```python
from build123d import *

# Parameters (mm, degrees)
CROQUIS1_W              = 37.6
CROQUIS1_H              = 15
CROQUIS1_R              = 1.5
SALIENTE_EXTRUIR1_DEPTH = 2
CROQUIS2_W              = 2.997393123
CROQUIS2_H              = 15
SALIENTE_EXTRUIR2_DEPTH = 20
CROQUIS3_R              = 1.3
CORTAR_EXTRUIR1_DEPTH   = 20


with BuildPart() as part:
    # Croquis1 → Saliente-Extruir1 (new body)
    with BuildSketch(Plane(origin=(0, 0, 0), x_dir=(1, 0, 0), z_dir=(0, 1, 0))):
        Rectangle(CROQUIS1_W, CROQUIS1_H)
        with Locations(Location((14.3, -3.2, 0), (0, 0, 270))):
            Circle(CROQUIS1_R, mode=Mode.SUBTRACT)
        with Locations(Location((-14.3, -3.2, 0), (0, 0, 90))):
            Circle(CROQUIS1_R, mode=Mode.SUBTRACT)
    extrude(amount=SALIENTE_EXTRUIR1_DEPTH)

    # Croquis2 → Saliente-Extruir2 (add)
    with BuildSketch(Plane(origin=(0, 2, 0), x_dir=(1, 0, 0), z_dir=(0, 1, 0))):
        with Locations((-4.748696562, 0)):
            Rectangle(CROQUIS2_W, CROQUIS2_H)
        with Locations((4.748696562, 0)):
            Rectangle(CROQUIS2_W, CROQUIS2_H)
    extrude(amount=SALIENTE_EXTRUIR2_DEPTH)

    # Croquis3 → Cortar-Extruir1 (cut)
    with BuildSketch(Plane.ZY.offset(6.247393123)):
        with Locations((0.3, 16.669676255)):
            Circle(CROQUIS3_R)
        with Locations((0.3, 7.330323745)):
            Circle(CROQUIS3_R)
    extrude(amount=-CORTAR_EXTRUIR1_DEPTH, mode=Mode.SUBTRACT)


solid = part.part
```
CAD build for the part. Positions are in the model's coordinates, mm. A direction names the side the tool comes from. Round coordinates to 2 decimals unless told otherwise and drop trailing zeros. Loops run counter-clockwise (first coordinate to the right, second up) from the corner with the lowest first, then second, coordinate; pieces in that order, holes last. Notation, with made-up numbers: M 49,53.5 L 100,53.5 A16 cw 100,68.5 Z; hole C 25.5,38 d7. An arc over 180 degrees is marked long. Use a Markdown table: item, result. Add a question column.
(1) Pull direction X, two halves, no side cores. Call faces 1 (the face through (6.247, 12, 0)), 2 (the face through (0, 2, 0)), 3 (the face through (12.836, 0.986, 2.875)), 4 (the face through (-4.77, 8.426, 0.999)): +X half, -X half, draft (parallel to the pull), parting line (faces both ways), or undercut.
(2) Cut at A-A (z = 3.2). Give the cut face in (x, y).
(3) Which spindle directions (+Z, -Z, +X, -X, +Y, -Y) get a long thin tool onto all of the face, cutting with end or side? Do faces 5 (the face through (-6.247, 12, 0)), 6 (the face through (3.25, 12, 0)), 7 (the face through (12, 2, 0)). Say none if no direction does.
(4) Cut at B-B (y = 13.75). Give the cut face in (x, z), and give its area (3 significant figures).
(5) Flat gauge pins, fed straight in: pin 1 (3 mm diameter, centred on y = 7.33, z = 0.3, fed in from +X); pin 2 (5 mm diameter, centred on x = 14.3, z = 3.2, fed in from -Y); pin 3 (3.5 mm diameter, centred on y = 16.67, z = 0.3, fed in from -X). Where does each tip first touch, or does it go through?
(6) Cut at C-C (x = 14.3). Give the cut face in (y, z).
(7) Cut at D-D (x = -4). Give the cut face in (y, z), and give its area (3 significant figures).
(8) Drill centre lines: line 1 (Y direction, x = -4.8, z = 0.3); line 2 (X direction, y = 11.5, z = -6.25); line 3 (Y direction, x = -4, z = 0.75). Where is each one in solid material? Low to high.
Geometry says:
| question | item | result |
|---|---|---|
| 1 | face 1 | +X half |
| 1 | face 2 | undercut |
| 1 | face 3 | undercut |
| 1 | face 4 | draft |
| 2 | outline | M -18.8,0 L -15.8,0 L -15.8,2 L -18.8,2 Z; M -12.8,0 L 12.8,0 L 12.8,2 L 6.25,2 L 6.25,22 L 3.25,22 L 3.25,2 L -3.25,2 L -3.25,22 L -6.25,22 L -6.25,2 L -12.8,2 Z; M 15.8,0 L 18.8,0 L 18.8,2 L 15.8,2 Z |
| 3 | face 5 | +Z, -Z, -X, +Y |
| 3 | face 6 | +Z, -Z, +Y |
| 3 | face 7 | +Z, -Z, +X, +Y |
| 4 | outline | M -6.25,-7.5 L -3.25,-7.5 L -3.25,7.5 L -6.25,7.5 Z; M 3.25,-7.5 L 6.25,-7.5 L 6.25,7.5 L 3.25,7.5 Z |
| 4 | area | 89.9 mm² |
| 5 | pin 1 | stops at x = 6.25 |
| 5 | pin 2 | stops at y = 0 |
| 5 | pin 3 | stops at x = -6.25 |
| 6 | outline | M 0,-7.5 L 2,-7.5 L 2,1.7 L 0,1.7 Z; M 0,4.7 L 2,4.7 L 2,7.5 L 0,7.5 Z |
| 7 | outline | M 0,-7.5 L 22,-7.5 L 22,7.5 L 0,7.5 Z; hole C 7.33,0.3 d2.6; hole C 16.67,0.3 d2.6 |
| 7 | area | 319 mm² |
| 8 | line 1 | y = 0 to 6.03, 8.63 to 15.37, 17.97 to 22 |
| 8 | line 2 | x = -6.25 to -3.25, 3.25 to 6.25 |
| 8 | line 3 | y = 0 to 6.11, 8.55 to 15.45, 17.89 to 22 |
